Autodesk Inventor part; units mm, degrees
ref_plane "Work Plane1" through (1.4732, 0, 0) normal (-1, 0, 0) x (0, 0, 1)
ref_plane "YZ Plane" through (0, 0, 0) normal (1, 0, 0) x (0, 1, 0)
ref_plane "XZ Plane" through (0, 0, 0) normal (0, 1, 0) x (-1, 0, 0)
sketch "Sketch1" plane through (0, 0, 0) normal (1, 0, 0) x (0, 1, 0)
  line L0 (0, 0) -> (0, -7.9426)
  line L1 (0, -7.9426) -> (3.236, -7.9426)
  line L2 (3.236, -7.9426) -> (3.236, -15.8852)
  line L3 (3.236, -15.8852) -> (6.4618, -15.8852)
  arc A0 (6.4618, -15.8852) -> (0, 0) centre (-13.924, -14.9208) ccw
  dimension "d0" = 7.9426
  dimension "d1" = 3.236
  dimension "d2" = 7.9426
  dimension "d3" = 3.2258
extrude "Extrusion1" add sketch "Sketch1" along normal blind 7.7978
shell "Shell1" thickness 1.4732 removed faces 1 at (2.5993, 0, -2.6475)
ref_plane "Work Plane1" through (1.4732, 0, 0) normal (-1, 0, 0) x (0, 0, 1)
sketch "Sketch4" plane through (1.4732, 0, 0) normal (-1, 0, 0) x (0, 0, 1)
  line L0 (-7.9426, 3.236) -> (-15.8852, 3.236)
  line L1 (-15.8852, 3.236) -> (-15.8852, 6.4618)
  arc A0 (0, 0) -> (-15.8852, 6.4618) centre (-14.9208, -13.924) ccw
  line L2 (-14.412, 4.7092) -> (-14.412, 5.0045)
  arc A1 (-7.9426, 3.6786) -> (-14.412, 5.0045) centre (-14.9208, -13.924) ccw
  line L3 (-14.412, 5.0045) -> (-14.412, 3.236)
  line L4 (-7.9426, 3.236) -> (-15.8852, 3.236)
  line L5 (-7.9426, 3.236) -> (-7.9426, 3.6786)
extrude "Extrusion2" cut sketch "Sketch4" against normal blind 4.8514
properties part number "2x1 curve" material "ABS Plastic"
Check sheet for the modelled part. Datum: model origin and axes. Units: mm. A direction names the side the tool comes from. Give positions to 0.01 mm unless a question says otherwise; leave off trailing zeros. Loops run counter-clockwise (first coordinate to the right, second up) from the corner with the lowest first, then second, coordinate; pieces in that order, holes last. Notation, with made-up numbers: M -35.75,42.25 L -17.75,42.25 A18 cw -17.75,61.25 Z; hole C -23,-9.75 d1. An arc over 180 degrees is marked long. Answer as CSV lines item,"result".
Item 1: Sectioned sample at C-C, the plane z = -10.75. Enter the section's corners in (x, y).
Reply:
outline,"M 0,3.24 L 1.47,3.24 L 1.47,4.55 L 6.32,4.55 L 6.32,3.24 L 7.8,3.24 L 7.8,6.05 L 0,6.05 Z"
Item 2: Draft check along Y on faces 4 (the face through (7.798, 4, -8)), 5 (the face through (3.844, 4.933, -7.116)), 6 (the face through (1, 0, -4)). Enter one of: pulls with the +Y half, pulls with the -Y half, needs draft (parallel to the pull), parting line crosses it, or undercut.
Reply:
face 4,"needs draft"
face 5,"pulls with the +Y half"
face 6,"pulls with the -Y half"
Item 3: Set-up check for faces 1 (the face through (4, 5, -15.885)), 2 (the face through (4, 3.236, -15)), 3 (the face through (1.473, 4, -12)): record each of +Z, -Z, +X, -X, +Y, -Y from which the full face is reachable in a straight line by a thin tool's end or side.
Reply:
face 1,"-Z, +X, -X, +Y, -Y"
face 2,"-Z, +X, -X, -Y"
face 3,"-Y"
Item 4: Sectioned sample at D-D, the plane y = 2.5. Enter the section's corners in (x, z).
Reply:
outline,"M 0,-7.94 L 7.8,-7.94 L 7.8,-2.81 L 0,-2.81 Z; hole M 1.47,-6.47 L 6.32,-6.47 L 6.32,-5.5 L 1.47,-5.5 Z"
Item 5: Sectioned sample at A-A, the plane x = 2.75. Enter the section's corners in (y, z).
Reply:
outline,"M 0,-7.94 L 3.68,-7.94 A18.94 cw 4.71,-11.55 A18.94 cw 5,-14.41 L 3.24,-14.41 L 3.24,-15.89 L 6.46,-15.89 A20.41 ccw 0,0 L 0,-2.09 A18.94 cw 3.02,-6.47 L 0,-6.47 Z"
Item 6: Sectioned sample at B-B, the plane y = 1.25. Enter the section's corners in (x, z), then the cut area to 3 significant figures.
Reply:
outline,"M 0,-7.94 L 7.8,-7.94 L 7.8,-1.27 L 0,-1.27 Z; hole M 1.47,-6.47 L 6.32,-6.47 L 6.32,-3.59 L 1.47,-3.59 Z"
area,"38.1 mm^2"
Item 7: Depth check by flat-ended pin: pin 1 Ø3 at (x, z) = (3.5, -3) entering from +Y; pin 2 Ø3.5 at (x, y) = (3.5, 1.5) entering from +Z; pin 3 Ø4 at (x, z) = (2.5, -10.5) entering from -Y. Enter the tip coordinate at first touch or a pass-through.
Reply:
pin 1,"y = 3.62"
pin 2,"z = 0"
pin 3,"y = 3.24"
Item 8: Scan lines: L1, parallel to Y at x = 7, z = -14; L2, parallel to Z at x = 2.25, y = 2.5; L3, parallel to Z at x = 5.5, y = 1.75. Record each from-to range of solid material in increasing order.
Reply:
L1,"3.24 to 6.46"
L2,"-7.94 to -6.47, -5.5 to -2.81"
L3,"-7.94 to -6.47, -4.3 to -1.85"
